Model file for the job. Use its own axes, mm. A direction names the side the tool comes from. Coordinates: 2 decimals unless noted, no trailing zeros. Write each loop counter-clockwise with the first axis right and the second up, starting at its lowest first coordinate (ties: lowest second). Pieces come first, ordered by that corner, then holes. Notation, with made-up numbers: (74, -1.5) -> (81, -1.5) arc R35 cw to (81, 34.5) -> close; hole circle Ø9 at (79, 70.5). An arc over 180 degrees is marked (long way). Answer as a JSON object with one key per item and string values. Group by question number.
from build123d import *

# Parameters (mm, degrees)
BODY_DEPTH      = 10
SHELL_START     = 3
SHELL_OUTLINE_W = 26
SHELL_OUTLINE_H = 14
SHELL_DEPTH     = 25


# Read off the part's stored shape, not the designer's step: Shell
with BuildPart() as part:
    # Sketch1 → Body (new, symmetric)
    with BuildSketch(Plane.XY):
        Polygon((28, 0), (0, 0), (0, 28), (3, 28), (28, 3), align=None)
    extrude(amount=BODY_DEPTH, both=True)

    # Shell outline → Shell (cut)
    with BuildSketch(Plane.YZ.offset(SHELL_START)):
        with Locations((16, 0)):
            Rectangle(SHELL_OUTLINE_W, SHELL_OUTLINE_H)
    extrude(amount=SHELL_DEPTH, mode=Mode.SUBTRACT)


solid = part.part
(1) 3-axis set-ups, long thin cutter, end or side, ignore diameter. For faces 1 (the face through (0, 14, 0)), 2 (the face through (15, 3, 0)): which of +Z, -Z, +X, -X, +Y, -Y reach the whole face in a straight line?
(2) Cut at C-C on z = -5. List the corners of the cut face in (x, y).
(3) Cut at A-A on x = 23.75. List the corners of the cut face in (y, z), plus the area to 3 significant figures.
(4) Pin check, flat tips, straight feed: pin 1 (7 mm diameter, centred on y = 12, z = 0.5, fed in from +X); pin 2 (1.5 mm diameter, centred on x = 21, z = 0.5, fed in from +Y). Stop position of each tip, or through.
(5) Wall check: probe 1 along Z at (x, y) = (16.5, 11.5); probe 2 along X at (y, z) = (5.25, 1.5). Give the ranges that are in metal, low to high.
(6) Cut at B-B on y = 5. List the corners of the cut face in (x, z).
(7) Pull direction Z, two halves, no side cores. Call faces 3 (the face through (13, 13, -7)), 4 (the face through (11, 11, 10)), 5 (the face through (14, 0, 0)): released by +Z, released by -Z, zero draft, split by the parting line, or undercut.
Results found:
{
 "1": {"face 1": "+Z, -Z, -X, +Y, -Y", "face 2": "+X, +Y"},
 "2": {"outline": "(0, 0) -> (28, 0) -> (28, 3) -> (3, 3) -> (3, 28) -> (0, 28) -> close"},
 "3": {"outline": "(0, -10) -> (7.25, -10) -> (7.25, -7) -> (3, -7) -> (3, 7) -> (7.25, 7) -> (7.25, 10) -> (0, 10) -> close", "area": "85.5 mm²"},
 "4": {"pin 1": "stops at x = 3", "pin 2": "stops at y = 3"},
 "5": {"probe 1": "z = -10 to -7, 7 to 10", "probe 2": "x = 0 to 3"},
 "6": {"outline": "(0, -10) -> (26, -10) -> (26, -7) -> (3, -7) -> (3, 7) -> (26, 7) -> (26, 10) -> (0, 10) -> close"},
 "7": {"face 3": "undercut", "face 4": "released by +Z", "face 5": "zero draft"}
}
